from build123d import *

# Parameters (mm, degrees)
F0_R     = 2
F1_DEPTH = 3
F2_SIZE2 = 2
F2_SIZE  = 4
F3_SIZE  = 0.5


with BuildPart() as f1:
    # F0 (on Top) → F1 (new body)
    with BuildSketch(Plane.XY):
        with BuildLine():
            ThreePointArc((-8.3460629921, 2.6278760495), (-3.05, 0), (-8.3460629921, -2.6278760495))
            ThreePointArc((-8.3460629921, -2.6278760495), (-6.1871843354, -6.1871843354), (-2.6278760495, -8.3460629921))
            ThreePointArc((-2.6278760495, -8.3460629921), (0, -3.05), (2.6278760495, -8.3460629921))
            ThreePointArc((2.6278760495, -8.3460629921), (6.1871843354, -6.1871843354), (8.3460629921, -2.6278760495))
            ThreePointArc((8.3460629921, -2.6278760495), (3.05, 0), (8.3460629921, 2.6278760495))
            ThreePointArc((8.3460629921, 2.6278760495), (6.1871843354, 6.1871843354), (2.6278760495, 8.3460629921))
            ThreePointArc((2.6278760495, 8.3460629921), (0, 3.05), (-2.6278760495, 8.3460629921))
            ThreePointArc((-2.6278760495, 8.3460629921), (-6.1871843354, 6.1871843354), (-8.3460629921, 2.6278760495))
        make_face()
        Circle(F0_R, mode=Mode.SUBTRACT)
    extrude(amount=F1_DEPTH)

    # F2
    f2_edges = [f1.edges().sort_by_distance(p)[0] for p in [
        (-6.187184, 6.187184, 3),
        (-6.187184, -6.187184, 3),
        (6.187184, -6.187184, 3),
        (6.187184, 6.187184, 3),
    ]]
    f2_side = f1.faces().sort_by_distance((-6.020263, 6.020263, 3))[0]
    chamfer(f2_edges, length=F2_SIZE, length2=F2_SIZE2, reference=f2_side)

    # F3
    f3_edges = [f1.edges().sort_by_distance(p)[0] for p in [
        (-2, 0, 3),
    ]]
    chamfer(f3_edges, length=F3_SIZE)


solid = f1.part
Could you check a few things on this model? Use its own coordinates, in mm. Give positions to 0.01 mm unless a question says otherwise; leave off trailing zeros. Order: outer loops, then holes, each group sorted by start corner. A loop starts at its lowest first (then second) coordinate and runs counter-clockwise, first axis right, second up.
1. I need wall thicknesses on L1, parallel to Y at x = 0, z = 0.65; L2, parallel to X at y = 4.25, z = 0.5; L3, parallel to X at y = -0.25, z = 0.3. Which ranges of each line are inside material? Lowest first, please.
2. Suppose I cut it at A-A (y = 0). List the corners of the cut face in (x, z) for me, plus the area to 3 significant figures.
3. We'd pull the mould along X, two halves only. Please class faces 1 (the conical face through (4.76, -4.82, 1.99)), 2 (the cylindrical face through (3.05, -0.1, 1.15)), 3 (the flat face through (2, 2, 3)), 4 (the cylindrical face through (-3.05, 0.1, 1.15)): pulls with the +X half, pulls with the -X half, needs draft (parallel to the pull), parting line crosses it, or undercut.
4. Suppose I cut it at B-B (z = 0.8). List the corners of the cut face in (x, y) for me, plus the area to 3 significant figures.
5. Will these pins go through, and if not, where does the flat tip stop? P1, Ø5.5, axis at x = -6.35, y = 0, coming from the +Z side (3 decimals); P2, Ø1.5, axis at x = 4, y = -4.5, coming from the +Z side; P3, Ø1, axis at x = -0.5, z = 1.5, coming from the +Y side.
Solved:
1. L1: y = -3.05 to -2, 2 to 3.05
1. L2: x = -7.65 to -2.55, 2.55 to 7.65
1. L3: x = -3.06 to -1.98, 1.98 to 3.06
2. outline: (-3.05, 0) - (-2, 0) - (-2, 2.5) - (-2.5, 3) - (-3.05, 3) - close; (2, 0) - (3.05, 0) - (3.05, 3) - (2.5, 3) - (2, 2.5) - close
2. area: 6.05 mm2
3. face 1: pulls with the +X half
3. face 2: undercut
3. face 3: needs draft
3. face 4: undercut
4. outline: (-8.35, -2.63) arc R8.75 ccw to (-2.63, -8.35) arc R3.3 cw (long way) to (2.63, -8.35) arc R8.75 ccw to (8.35, -2.63) arc R3.3 cw (long way) to (8.35, 2.63) arc R8.75 ccw to (2.63, 8.35) arc R3.3 cw (long way) to (-2.63, 8.35) arc R8.75 ccw to (-8.35, 2.63) arc R3.3 cw (long way) to start; hole circle Ø4 at (0, 0)
4. area: 105 mm2
5. P1: passes through
5. P2: stops at z = 2.74
5. P3: stops at y = 3.21
